Part model, mm, in its own coordinate system. Face numbers are marked on the shaded views. A direction names the side the tool comes from. Coordinates: 2 decimals unless noted, no trailing zeros. Write each loop counter-clockwise with the first axis right and the second up, starting at its lowest first coordinate (ties: lowest second). Pieces come first, ordered by that corner, then holes. Notation, with made-up numbers: (10.5, 72.25) - (29.5, 72.25) arc R29 cw to (29.5, 104.25) - close; hole circle Ø2 at (20, 15.5). An arc over 180 degrees is marked (long way). Use one line per item in the form item = value. Start each with the question number.
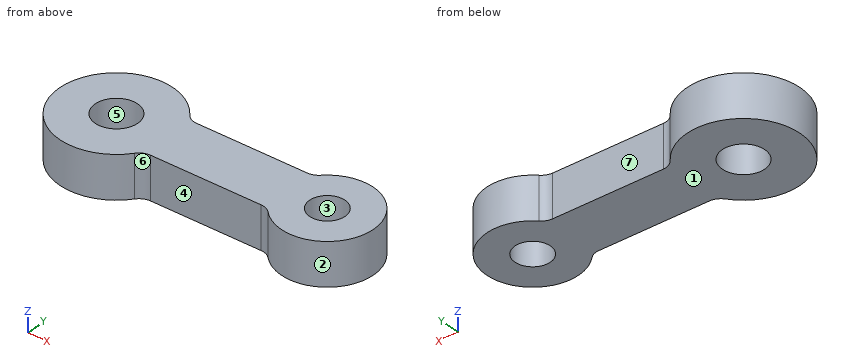
from build123d import *

# Parameters (mm, degrees)
ESQUISSE1_R        = 3
ESQUISSE1_R_2      = 2.5
BOSS_EXTRU_1_DEPTH = 6
CONG_1_R           = 2


with BuildPart() as part:
    # Esquisse1 → Boss.-Extru.1 (new body)
    with BuildSketch(Plane.XY):
        with BuildLine():
            Line((6.92820323, 4), (24.376524617, 4))
            ThreePointArc((24.376524617, 4), (36, 0), (24.376524617, -4))
            Line((24.376524617, -4), (6.92820323, -4))
            ThreePointArc((6.92820323, -4), (-8, 0), (6.92820323, 4))
        make_face()
        Circle(ESQUISSE1_R, mode=Mode.SUBTRACT)
        with Locations((29.5, 0)):
            Circle(ESQUISSE1_R_2, mode=Mode.SUBTRACT)
    extrude(amount=BOSS_EXTRU_1_DEPTH)

    # Congé1
    cong_1_edges = [part.edges().sort_by_distance(p)[0] for p in [
        (6.92820323, 4, 3),
        (24.376524617, 4, 3),
        (24.376524617, -4, 3),
        (6.92820323, -4, 3),
    ]]
    fillet(cong_1_edges, radius=CONG_1_R)


solid = part.part
Q1. Which spindle directions (+Z, -Z, +X, -X, +Y, -Y) get a long thin tool onto all of the face, cutting with end or side? Do the marked faces 5, 6 and 7. Say none if no direction does.
Q2. Slice it at C-C (y = 0). List the corners of the cut face in (x, z).
Q3. Mould opens along Y. For the marked faces 1, 2, 3 and 4 say: released by +Y, released by -Y, zero draft, split by the parting line, or undercut.
Q4. Slice it at A-A (x = 0). List the corners of the cut face in (y, z), plus the area to 3 significant figures.
Q5. Slice it at D-D (x = 29.5). List the corners of the cut face in (y, z).
Q6. Pin check, flat tips, straight feed: P1, Ø1.5, axis at y = 3, z = 3, coming from the -X side; P2, Ø2, axis at x = -1.5, z = 1.5, coming from the -Y side. Stop position of each tip, or through.
Q7. Drill centre lines: probe 1 along Y at (x, z) = (29.5, 2.3); probe 2 along Y at (x, z) = (0, 4.75); probe 3 along X at (y, z) = (-1.75, 0.5). Where is each one in solid material? Low to high.
Q8. Slice it at B-B (z = 4.5). List the corners of the cut face in (x, y), plus the area to 3 significant figures.
Solution:
q1.face_5 = +Z, -Z
q1.face_6 = +Z, -Z, -Y
q1.face_7 = +Z, -Z, +Y
q2.outline = (-8, 0) - (-3, 0) - (-3, 6) - (-8, 6) - close; (3, 0) - (27, 0) - (27, 6) - (3, 6) - close; (32, 0) - (36, 0) - (36, 6) - (32, 6) - close
q3.face_1 = zero draft
q3.face_2 = split by the parting line
q3.face_3 = undercut
q3.face_4 = released by -Y
q4.outline = (-8, 0) - (-3, 0) - (-3, 6) - (-8, 6) - close; (3, 0) - (8, 0) - (8, 6) - (3, 6) - close
q4.area = 60.0 mm2
q5.outline = (-6.5, 0) - (-2.5, 0) - (-2.5, 6) - (-6.5, 6) - close; (2.5, 0) - (6.5, 0) - (6.5, 6) - (2.5, 6) - close
q6.P1 = -7.68
q6.P2 = -7.98
q7.probe_1 = -6.5 to -2.5, 2.5 to 6.5
q7.probe_2 = -8 to -3, 3 to 8
q7.probe_3 = -7.81 to -2.44, 2.44 to 27.71, 31.29 to 35.76
q8.outline = (6.4, -4.8) arc R2 cw to (8, -4) - (23.48, -4) arc R2 cw to (24.9, -4.59) arc R6.5 ccw (long way) to (24.9, 4.59) arc R2 cw to (23.48, 4) - (8, 4) arc R2 cw to (6.4, 4.8) arc R8 ccw (long way) to start; hole circle Ø6 at (0, 0); hole circle Ø5 at (29.5, 0)
q8.area = 413 mm2
